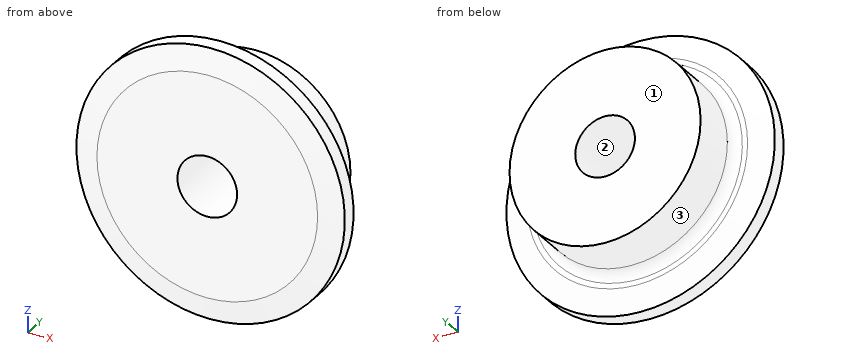
```python
from build123d import *

# Parameters (mm, degrees)
F0_W     = 5.91
F0_H     = 6.875
F0_W_2   = 2.84
F0_H_2   = 4.05
F2_R     = 1
F3_SIZE2 = 2.5
F3_SIZE  = 0.62


with BuildPart() as f1:
    # F0 (on Right) → F1 (revolve)
    with BuildSketch(Plane.YZ):
        with Locations((5.795, 6.5625)):
            Rectangle(F0_W, F0_H)
        with Locations((1.42, 6.5625)):
            Rectangle(F0_W_2, F0_H)
        with Locations((1.42, 12.025)):
            Rectangle(F0_W_2, F0_H_2)
    revolve(axis=Axis((0, 4.375, 0), (0, 1, 0)))

    # F2
    f2_edges = [f1.edges().sort_by_distance(p)[0] for p in [
        (0, 2.84, -10),
    ]]
    fillet(f2_edges, radius=F2_R)

    # F3
    f3_edges = [f1.edges().sort_by_distance(p)[0] for p in [
        (0, 0, -14.05),
        (0, 2.84, -14.05),
    ]]
    f3_side = f1.faces().sort_by_distance((0, 1.42, -14.05))[0]
    chamfer(f3_edges, length=F3_SIZE, length2=F3_SIZE2, reference=f3_side)


solid = f1.part
```
Geometry: final body of the model. Coordinates: model frame, mm. Face numbers are marked on the shaded views. Round coordinates to 2 decimals unless told otherwise and drop trailing zeros. Loops run counter-clockwise (first coordinate to the right, second up) from the corner with the lowest first, then second, coordinate; pieces in that order, holes last.
Item 1: Line query: L1, parallel to X at y = 6.75, z = 0 (3 decimals); L2, parallel to X at y = 1.5, z = 0 (3 decimals); L3, parallel to Y at x = -10.25, z = 5. Output: solid intervals per line, ascending.
Checked values:
L1: x = -10 to -3.125, 3.125 to 10
L2: x = -14.05 to -3.125, 3.125 to 14.05
L3: y = 0 to 2.84
Item 2: Contact query for flat-ended pins moving along their axis: P1, Ø1, axis at x = -4, y = 7, coming from the -Z side; P2, Ø4, axis at x = 6.5, y = 4, coming from the -Z side; P3, Ø1.5, axis at x = -7.5, z = 2.5, coming from the -Y side; P4, Ø5, axis at x = 0, z = 0, coming from the -Y side. Output: stop coordinate, or through.
Checked values:
P1: stops at z = -9.37
P2: stops at z = -12.89
P3: stops at y = 0
P4: passes through
Item 3: Section A-A, the plane x = 0. Output: boundary loops of the cut face in (y, z) (3 decimals), plus the area to 3 significant figures.
Checked values:
outline: (0, -11.55) - (0.62, -14.05) - (2.22, -14.05) - (2.84, -11.55) - (2.84, -11) arc R1 cw to (3.84, -10) - (8.75, -10) - (8.75, -3.125) - (0, -3.125) - close; (0, 3.125) - (8.75, 3.125) - (8.75, 10) - (3.84, 10) arc R1 cw to (2.84, 11) - (2.84, 11.55) - (2.22, 14.05) - (0.62, 14.05) - (0, 11.55) - close
area: 141 mm2
Item 4: Section D-D, the plane y = 5.5. Output: boundary loops of the cut face in (x, z) (3 decimals), plus the area to 3 significant figures.
Checked values:
outline: circle Ø20 at (0, 0); hole circle Ø6.25 at (0, 0)
area: 283 mm2
Item 5: Section B-B, the plane z = 0. Output: boundary loops of the cut face in (x, y) (3 decimals), plus the area to 3 significant figures.
Checked values:
outline: (-14.05, 0.62) - (-11.55, 0) - (-3.125, 0) - (-3.125, 8.75) - (-10, 8.75) - (-10, 3.84) arc R1 cw to (-11, 2.84) - (-11.55, 2.84) - (-14.05, 2.22) - close; (3.125, 0) - (11.55, 0) - (14.05, 0.62) - (14.05, 2.22) - (11.55, 2.84) - (11, 2.84) arc R1 cw to (10, 3.84) - (10, 8.75) - (3.125, 8.75) - close
area: 141 mm2
Item 6: Mould query, pull axis X, two halves, no side actions, for the marked faces 1, 2 and 3. Classes: released by +X, released by -X, zero draft, split by the parting line, or undercut.
Checked values:
face 1: zero draft
face 2: undercut
face 3: split by the parting line
Item 7: Section C-C, the plane y = 1. Output: boundary loops of the cut face in (x, z) (3 decimals), plus the area to 3 significant figures.
Checked values:
outline: circle Ø28.1 at (0, 0); hole circle Ø6.25 at (0, 0)
area: 589 mm2
